Verification items for this drawing (mm, ordinates from the low corner). Round coordinates to 2 decimals unless told otherwise and drop trailing zeros. Order: outer loops, then holes, each group sorted by start corner. A loop starts at its lowest first (then second) coordinate and runs counter-clockwise, first axis right, second up. Notation, with made-up numbers: (64.25, -5) -> (93.25, -5) arc R8 ccw to (93.25, 10) -> close; hole circle Ø2 at (84, 4.25). An arc over 180 degrees is marked (long way). Put each result on its own line as item: value.
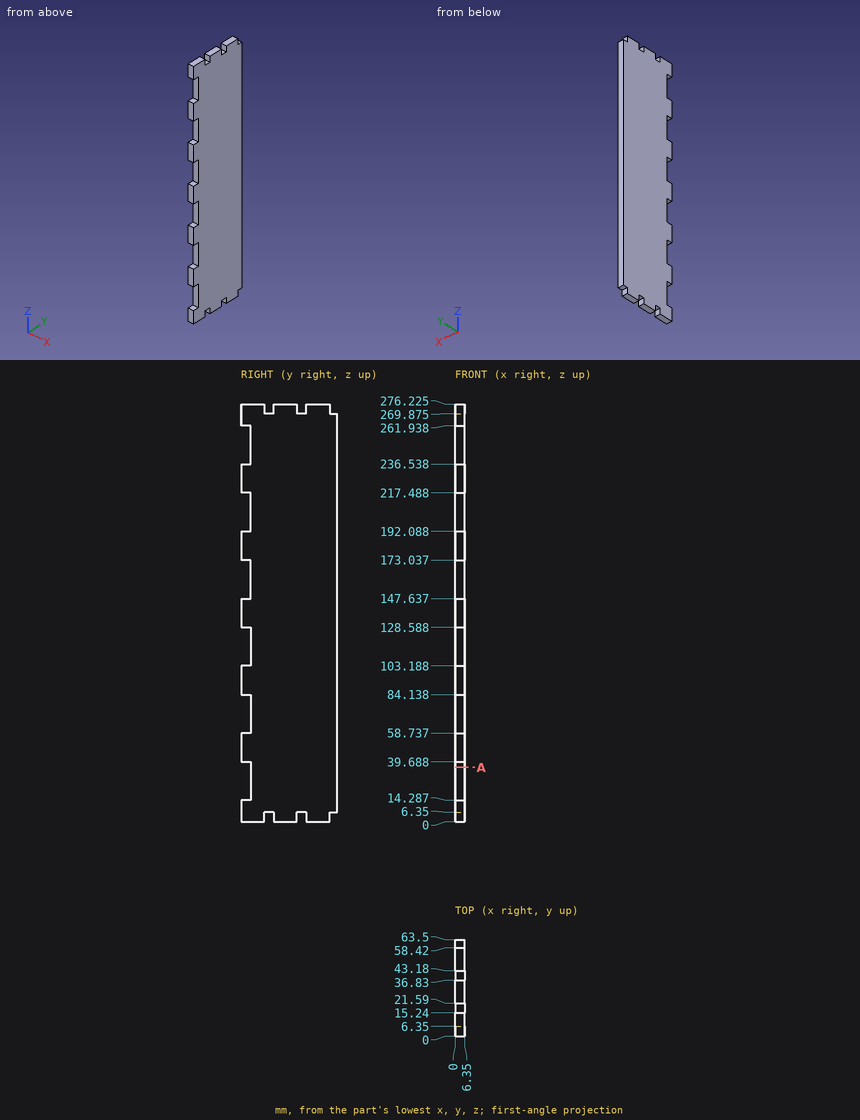
Item 1: Section check A-A on z = 36. Record the boundary of the cut face in (x, y).
Check sheet entries:
outline: (0, 6.35) -> (6.35, 6.35) -> (6.35, 63.5) -> (0, 63.5) -> close
Item 2: Material ranges on L1, parallel to Y at x = 2.5, z = 106, recorded low to high. Write a range as [from, to].
Check sheet entries:
L1: y = [6.35, 63.5]
Item 3: Gauge pin test, flat ends, axial feed: pin 1 Ø1.9 at (x, y) = (4.5, 3) entering from -Z; pin 2 Ø1.9 at (x, y) = (3, 39.5) entering from +Z (1 decimal); pin 3 Ø1.5 at (x, z) = (5, 121) entering from -Y; pin 4 Ø3 at (x, z) = (3, 273) entering from +Y. Record the tip position at first contact, or that the pin passes through.
Check sheet entries:
pin 1: stops at z = 0
pin 2: stops at z = 269.9
pin 3: stops at y = 6.35
pin 4: stops at y = 58.42
